Read the model definition and answer for the solid it produces. Units are mm, in the model's axes. Face numbers are marked on the shaded views. Coordinates: 2 decimals unless noted, no trailing zeros. Loops run counter-clockwise (first coordinate to the right, second up) from the corner with the lowest first, then second, coordinate; pieces in that order, holes last.
from build123d import *

# Parameters (mm, degrees)
PAD002_DEPTH  = 0.3
SKETCH_W      = 12.3
SKETCH_H      = 7.3
PAD_DEPTH     = 9.5
POCKET_DEPTH  = 0.25
CHAMFER_SIZE  = 0.24
FILLET_R      = 0.15
SKETCH001_W   = 0.5
SKETCH001_H   = 0.5
SKETCH001_W_2 = 0.3
SKETCH001_H_2 = 0.3
PAD001_DEPTH  = 4
PAD003_DEPTH  = 0.3


with BuildPart() as pad002:
    # Sketch003 → Pad002 (new body)
    with BuildSketch(Plane.YZ.offset(6.19)):
        with BuildLine():
            ThreePointArc((-10.21, 1.27), (-8.94, 0), (-7.67, 1.27))
            Line((-10.21, 1.27), (-7.67, 1.27))
        make_face()
        with BuildLine():
            ThreePointArc((-2.54, 1.27), (-1.27, 0), (0, 1.27))
            Line((-2.54, 1.27), (0, 1.27))
        make_face()
    extrude(amount=-PAD002_DEPTH)


with BuildPart() as fillet_body:
    # Sketch → Pad (new body)
    with BuildSketch(Plane(origin=(0, 0, 0.5), x_dir=(0, -1, 0), z_dir=(0, 0, 1))):
        with Locations((5.08, 2.54)):
            Rectangle(SKETCH_W, SKETCH_H)
    extrude(amount=PAD_DEPTH)

    # Sketch002 → Pocket (cut)
    with BuildSketch(Plane(origin=(0, 0, 10), x_dir=(0, -1, 0), z_dir=(0, 0, 1))):
        with BuildLine():
            ThreePointArc((-0.57, 4.69), (0.137107, 4.982894), (0.43, 5.690001))
            Line((0.43, 6.19), (0.43, 5.690001))
            Line((-1.07, 6.19), (0.43, 6.19))
            Line((-1.07, 4.69), (-1.07, 6.19))
            Line((-0.57, 4.69), (-1.07, 4.69))
        make_face()
    extrude(amount=-POCKET_DEPTH, mode=Mode.SUBTRACT)

    # Chamfer
    chamfer_edges = [fillet_body.edges().sort_by_distance(p)[0] for p in [
        (4.982894, -0.137107, 10),
        (5.940001, -0.43, 10),
        (4.69, 0.82, 10),
    ]]
    chamfer(chamfer_edges, length=CHAMFER_SIZE)

    # Fillet
    fillet_edges = [fillet_body.edges().sort_by_distance(p)[0] for p in [
        (6.19, -5.95, 10),
        (1.67, 1.07, 10),
        (-1.11, -5.08, 10),
        (2.54, -11.23, 10),
    ]]
    fillet(fillet_edges, radius=FILLET_R)


with BuildPart() as pad001:
    # Sketch001 → Pad001 (new body)
    with BuildSketch(Plane(origin=(0, 0, 0.6), x_dir=(0, -1, 0), z_dir=(0, 0, 1))):
        Rectangle(SKETCH001_W, SKETCH001_H)
        with Locations((2.64, 0)):
            Rectangle(SKETCH001_W_2, SKETCH001_H_2)
        with Locations((0, 5.08)):
            Rectangle(SKETCH001_W, SKETCH001_H)
        with Locations((2.64, 5.08)):
            Rectangle(SKETCH001_W_2, SKETCH001_H_2)
        with Locations((10.26, 0)):
            Rectangle(SKETCH001_W_2, SKETCH001_H_2)
        with Locations((10.26, 5.08)):
            Rectangle(SKETCH001_W_2, SKETCH001_H_2)
    extrude(amount=-PAD001_DEPTH)


with BuildPart() as obj1:
    # Sketch004 → Pad003 (new body)
    with BuildSketch(Plane.YZ.offset(-1.11)):
        with BuildLine():
            ThreePointArc((-10.21, 1.27), (-8.94, 0), (-7.67, 1.27))
            Line((-10.21, 1.27), (-7.67, 1.27))
        make_face()
        with BuildLine():
            ThreePointArc((-2.54, 1.27), (-1.27, 0), (0, 1.27))
            Line((-2.54, 1.27), (0, 1.27))
        make_face()
    extrude(amount=PAD003_DEPTH)

    # obj1: union Pad002, Fillet body, Pad001
    add(pad002.part)
    add(fillet_body.part)
    add(pad001.part)


solid = obj1.part
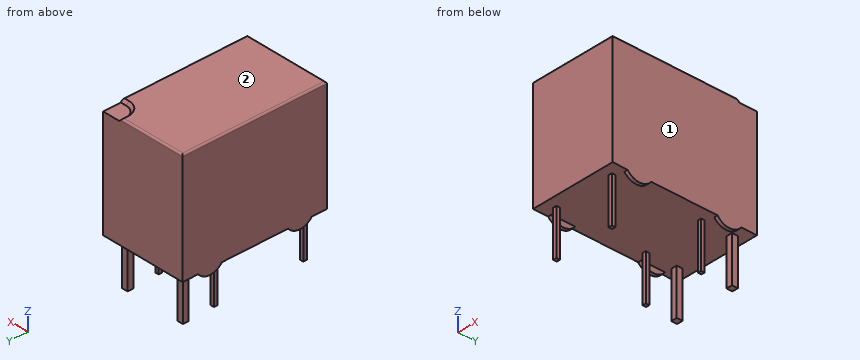
Q1. A cutting plane is placed at A-A (x = 1.25). Give the vertices of the cut face in (y, z).
Findings below:
outline: (-11.23, 0.5) - (1.07, 0.5) - (1.07, 9.85) arc R0.15 ccw to (0.92, 10) - (-11.08, 10) arc R0.15 ccw to (-11.23, 9.85) - close
Q2. Flat-ended cylindrical pins translate along their axes: pin 1 Ø0.6 at (x, z) = (5, -2) entering from +Y; pin 2 Ø3 at (x, y) = (2.5, -3.5) entering from -Z. Find the tip coordinate at first contact, or state that the pin passes through.
Findings below:
pin 1: stops at y = 0.25
pin 2: stops at z = 0.5
Q3. Determine the mould class of the marked faces 1 and 2 for opening direction Z: +Z half, -Z half, draft (parallel to the pull), parting line (faces both ways), or undercut.
Findings below:
face 1: draft
face 2: +Z half
Q4. A cutting plane is placed at C-C (y = -8.75). Give the vertices of the cut face in (x, z).
Findings below:
outline: (-1.11, 0.01) - (-0.81, 0.01) - (-0.81, 0.5) - (5.89, 0.5) - (5.89, 0.01) - (6.19, 0.01) - (6.19, 9.85) arc R0.15 ccw to (6.04, 10) - (-0.96, 10) arc R0.15 ccw to (-1.11, 9.85) - close
Q5. A cutting plane is placed at B-B (y = -5). Give the vertices of the cut face in (x, z).
Findings below:
outline: (-1.11, 0.5) - (6.19, 0.5) - (6.19, 9.85) arc R0.15 ccw to (6.04, 10) - (-0.96, 10) arc R0.15 ccw to (-1.11, 9.85) - close
Q6. Straight lines are drawn through the part: probe 1 along X at (y, z) = (0, -2.5); probe 2 along Z at (x, y) = (2, -0.75); probe 3 along Z at (x, y) = (5.5, 0). For each, find the intervals that lie inside material, in ascending order.
Findings below:
probe 1: x = -0.25 to 0.25, 4.83 to 5.33
probe 2: z = 0.5 to 10
probe 3: z = 0.5 to 9.75
